```python
from build123d import *

# Parameters (mm, degrees)
EXTRUDE_1_DEPTH     = 210
SKETCH_2_R          = 1.5
CUT_EXTRUDE_1_DEPTH = 10
SKETCH_3_R          = 1.5
CUT_EXTRUDE_2_DEPTH = 10
SKETCH_5_R          = 2.5
CUT_EXTRUDE_3_DEPTH = 10


with BuildPart() as part:
    # 草图1 → 凸台-拉伸1 (new body)
    with BuildSketch(Plane.XY):
        Polygon((2.52173913, 3.673913043), (4.52173913, 3.673913043), (4.52173913, -6.326086957), (-5.47826087, -6.326086957), (-5.47826087, 3.673913043), (-3.47826087, 3.673913043), (-3.47826087, -4.326086957), (2.52173913, -4.326086957), align=None)
    extrude(amount=EXTRUDE_1_DEPTH)

    # 草图2 → 切除-拉伸1 (cut)
    with BuildSketch(Plane(origin=(4.52173913, 0, 0), x_dir=(0, 0, -1), z_dir=(1, 0, 0))):
        with Locations(Location((-160, 0.673913043, 0), (0, 0, 90))):
            Circle(SKETCH_2_R)
        with Locations(Location((-135, 0.673913043, 0), (0, 0, 90))):
            Circle(SKETCH_2_R)
        with Locations(Location((-75, 0.673913043, 0), (0, 0, 90))):
            Circle(SKETCH_2_R)
        with Locations(Location((-50, 0.673913043, 0), (0, 0, 90))):
            Circle(SKETCH_2_R)
    extrude(amount=-CUT_EXTRUDE_1_DEPTH, mode=Mode.SUBTRACT)

    # 草图3 → 切除-拉伸2 (cut)
    with BuildSketch(Plane(origin=(4.52173913, 0, 0), x_dir=(0, 0, -1), z_dir=(1, 0, 0))):
        with Locations(Location((-20, -1.326086957, 0), (0, 0, 90))):
            Circle(SKETCH_3_R)
        with Locations(Location((-190, -1.326086957, 0), (0, 0, 90))):
            Circle(SKETCH_3_R)
    extrude(amount=-CUT_EXTRUDE_2_DEPTH, mode=Mode.SUBTRACT)

    # 草图5 → 切除-拉伸3 (cut)
    with BuildSketch(Plane.XZ.offset(6.326086957)):
        with Locations((-0.47826087, 105)):
            Circle(SKETCH_5_R)
    extrude(amount=-CUT_EXTRUDE_3_DEPTH, mode=Mode.SUBTRACT)


solid = part.part
```
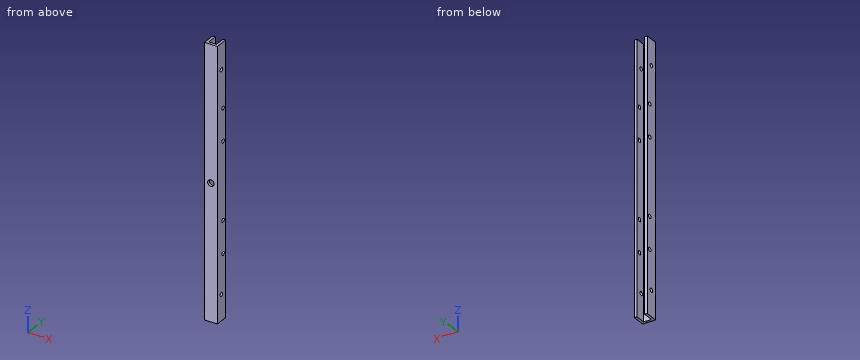
Input: part model. Units: mm. Frame: model coordinates. Give positions to 0.01 mm unless a question says otherwise; leave off trailing zeros. Write each loop counter-clockwise with the first axis right and the second up, starting at its lowest first coordinate (ties: lowest second). Pieces come first, ordered by that corner, then holes. Notation, with made-up numbers: (-3.75, 66) - (31.25, 66) arc R24 cw to (31.25, 93) - close; hole circle Ø10 at (-0.5, 46). An arc over 180 degrees is marked (long way). Write item = value, one per line. Start each with the question number.
1. Section query B-B, the plane x = 0. Output: boundary loops of the cut face in (y, z).
2. Section query A-A, the plane z = 182.5. Output: boundary loops of the cut face in (x, y), then the cut area to 3 significant figures.
3. Ray query, L1, parallel to Y at x = 3.2, z = 190; L2, parallel to X at y = -3.75, z = 136; L3, parallel to Y at x = -4.25, z = 135. Return the intervals inside material, ascending.
Check sheet entries:
q1.outline = (-6.33, 0) - (-4.33, 0) - (-4.33, 102.55) - (-6.33, 102.55) - close; (-6.33, 107.45) - (-4.33, 107.45) - (-4.33, 210) - (-6.33, 210) - close
q2.outline = (-5.48, -6.33) - (4.52, -6.33) - (4.52, 3.67) - (2.52, 3.67) - (2.52, -4.33) - (-3.48, -4.33) - (-3.48, 3.67) - (-5.48, 3.67) - close
q2.area = 52.0 mm2
q3.L1 = -6.33 to -2.83, 0.17 to 3.67
q3.L2 = -5.48 to -3.48, 2.52 to 4.52
q3.L3 = -6.33 to -0.83, 2.17 to 3.67
